from build123d import *

# Parameters (mm, degrees)
F0_W     = 115
F0_H     = 84
F1_DEPTH = 25
F2_T     = -2
F3_R     = 10
F4_W     = 19.5
F4_H     = 27.5
F5_DEPTH = 25
F6_W     = 4.8
F6_H     = 15
F7_DEPTH = 84.001
F8_W     = 15
F8_H     = 4.286
F9_DEPTH = 25


with BuildPart() as f1:
    # F0 (on Front) → F1 (new body)
    with BuildSketch(Plane.XZ):
        with Locations((-91.9387002908, -17.9252284579)):
            Rectangle(F0_W, F0_H)
    extrude(amount=F1_DEPTH)

    # F2
    f2_openings = [f1.faces().sort_by_distance(p)[0] for p in [
        (-91.9387, -25, -17.925228),
        (-149.4387, -12.5, -17.925228),
    ]]
    offset(amount=F2_T, openings=f2_openings)

    # F3
    f3_edges = [f1.edges().sort_by_distance(p)[0] for p in [
        (-149.4387, -25, 23.074772),
        (-149.4387, -25, -58.925228),
    ]]
    fillet(f3_edges, radius=F3_R)

    # F4 (on face) → F5 (cut)
    with BuildSketch(Plane(origin=(0, 0, 0), x_dir=(-1, 0, 0), z_dir=(0, 1, 0))):
        with Locations((56.1887002908, -1.6752284579)):
            Rectangle(F4_W, F4_H)
        with Locations((80.6887002908, -1.6752284579)):
            Rectangle(F4_W, F4_H)
        with Locations((105.1887002908, -1.6752284579)):
            Rectangle(F4_W, F4_H)
        with Locations((129.6887002908, -1.6752284579)):
            Rectangle(F4_W, F4_H)
        with Locations((129.6887002908, -34.1752284579)):
            Rectangle(F4_W, F4_H)
        with Locations((105.1887002908, -34.1752284579)):
            Rectangle(F4_W, F4_H)
        with Locations((80.6887002908, -34.1752284579)):
            Rectangle(F4_W, F4_H)
        with Locations((56.1887002908, -34.1752284579)):
            Rectangle(F4_W, F4_H)
    extrude(amount=-F5_DEPTH, mode=Mode.SUBTRACT)

    # F6 (on face) → F7 (cut, through all)
    with BuildSketch(Plane.XY.offset(24.0747715421)):
        with Locations((-48.8387002908, -12.5)):
            Rectangle(F6_W, F6_H)
        with Locations((-58.6387002908, -12.5)):
            Rectangle(F6_W, F6_H)
        with Locations((-68.4387002908, -12.5)):
            Rectangle(F6_W, F6_H)
        with Locations((-78.2387002908, -12.5)):
            Rectangle(F6_W, F6_H)
        with Locations((-88.0387002908, -12.5)):
            Rectangle(F6_W, F6_H)
        with Locations((-97.8387002908, -12.5)):
            Rectangle(F6_W, F6_H)
        with Locations((-107.6387002908, -12.5)):
            Rectangle(F6_W, F6_H)
        with Locations((-117.4387002908, -12.5)):
            Rectangle(F6_W, F6_H)
        with Locations((-127.2387002908, -12.5)):
            Rectangle(F6_W, F6_H)
        with Locations((-137.0387002908, -12.5)):
            Rectangle(F6_W, F6_H)
    extrude(amount=-F7_DEPTH, mode=Mode.SUBTRACT)

    # F8 (on face) → F9 (cut)
    with BuildSketch(Plane.YZ.offset(-34.4387002908)):
        with Locations((-12.5, -45.7822284579)):
            Rectangle(F8_W, F8_H)
        with Locations((-12.5, -36.4965141579)):
            Rectangle(F8_W, F8_H)
        with Locations((-12.5, -27.2107998579)):
            Rectangle(F8_W, F8_H)
        with Locations((-12.5, -17.9250855579)):
            Rectangle(F8_W, F8_H)
        with Locations((-12.5, -8.6393712579)):
            Rectangle(F8_W, F8_H)
        with Locations((-12.5, 0.6463430421)):
            Rectangle(F8_W, F8_H)
        with Locations((-12.5, 9.9320573421)):
            Rectangle(F8_W, F8_H)
    extrude(amount=-F9_DEPTH, mode=Mode.SUBTRACT)


solid = f1.part
Work out the finished part from the listing and answer in its coordinate system (mm). A direction names the side the tool comes from. Give positions to 0.01 mm unless a question says otherwise; leave off trailing zeros. Write each loop counter-clockwise with the first axis right and the second up, starting at its lowest first coordinate (ties: lowest second). Pieces come first, ordered by that corner, then holes. Notation, with made-up numbers: (-33.5, -20.75) - (1.5, -20.75) arc R21 ccw to (1.5, -2.75) - close; hole circle Ø10 at (4, -14). An arc over 180 degrees is marked (long way). One line per item, written item: value. Start each with the question number.
1. Find section D-D (y = -3.5). Write down the section's boundary in (x, z), then the cut area to 3 significant figures.
2. Find section B-B (x = -127). Write down the section's boundary in (y, z).
3. For faces 5 (the flat face through (-34.439, -21, -19)), 6 (the flat face through (-36.439, -21, -18)), determine the directions among +Z, -Z, +X, -X, +Y, -Y from which every point of the face is accessible in a straight line to the end or side of a thin tool.
4. For a pull along Z with two mould halves and no side action, classify faces 1 (the flat face through (-94, -2, -17)), 2 (the flat face through (-93, -12, -59.925)), 3 (the flat face through (-87.2, -25, -58.2)), 4 (the flat face through (-94, -13, -57.925)) as +Z half, -Z half, draft (parallel to the pull), parting line (faces both ways), or undercut.
5. Given pin 1 (1.5 mm diameter, centred on y = -14.5, z = -11, fed in from -X), flat-ended and moving along its own axis, determine where the tip first touches the part or whether it passes through.
6. Find section C-C (z = -40). Write down the section's boundary in (x, y).
7. Find section A-A (z = -27.5). Write down the section's boundary in (x, y), then the cut area to 3 significant figures.
8. Consider probe 1 along X at (y, z) = (-1, -44); probe 2 along Z at (x, y) = (-114.5, -9.5); probe 3 along X at (y, z) = (-10.75, -42.5). Determine where each line is inside the solid, lowest interval first.
Geometry results:
1. outline: (-149.44, -59.93) - (-34.44, -59.93) - (-34.44, 24.07) - (-149.44, 24.07) - (-149.44, 22.07) - (-36.44, 22.07) - (-36.44, -57.93) - (-149.44, -57.93) - close
1. area: 620 mm2
2. outline: (-25, -59.93) - (-20, -59.93) - (-20, -57.93) - (-25, -57.93) - close; (-25, 22.07) - (-20, 22.07) - (-20, 24.07) - (-25, 24.07) - close; (-5, -59.93) - (0, -59.93) - (0, -47.93) - (-2, -47.93) - (-2, -57.93) - (-5, -57.93) - close; (-5, 22.07) - (-2, 22.07) - (-2, 12.07) - (0, 12.07) - (0, 24.07) - (-5, 24.07) - close; (-2, -20.43) - (0, -20.43) - (0, -15.43) - (-2, -15.43) - close
3. face 5: +Z, -Z, +X, +Y, -Y
3. face 6: -X, -Y
4. face 1: undercut
4. face 2: -Z half
4. face 3: draft
4. face 4: undercut
5. pin 1: x = -36.44
6. outline: (-149.44, -2) - (-139.44, -2) - (-139.44, 0) - (-149.44, 0) - close; (-119.94, -2) - (-114.94, -2) - (-114.94, 0) - (-119.94, 0) - close; (-95.44, -2) - (-90.44, -2) - (-90.44, 0) - (-95.44, 0) - close; (-70.94, -2) - (-65.94, -2) - (-65.94, 0) - (-70.94, 0) - close; (-46.44, -2) - (-36.44, -2) - (-36.44, -25) - (-34.44, -25) - (-34.44, 0) - (-46.44, 0) - close
7. outline: (-149.44, -2) - (-139.44, -2) - (-139.44, 0) - (-149.44, 0) - close; (-119.94, -2) - (-114.94, -2) - (-114.94, 0) - (-119.94, 0) - close; (-95.44, -2) - (-90.44, -2) - (-90.44, 0) - (-95.44, 0) - close; (-70.94, -2) - (-65.94, -2) - (-65.94, 0) - (-70.94, 0) - close; (-46.44, -2) - (-36.44, -2) - (-36.44, -5) - (-34.44, -5) - (-34.44, 0) - (-46.44, 0) - close; (-36.44, -25) - (-34.44, -25) - (-34.44, -20) - (-36.44, -20) - close
7. area: 90.0 mm2
8. probe 1: -149.44 to -139.44, -119.94 to -114.94, -95.44 to -90.44, -70.94 to -65.94, -46.44 to -34.44
8. probe 2: -59.93 to -57.93, 22.07 to 24.07
8. probe 3: -36.44 to -34.44
